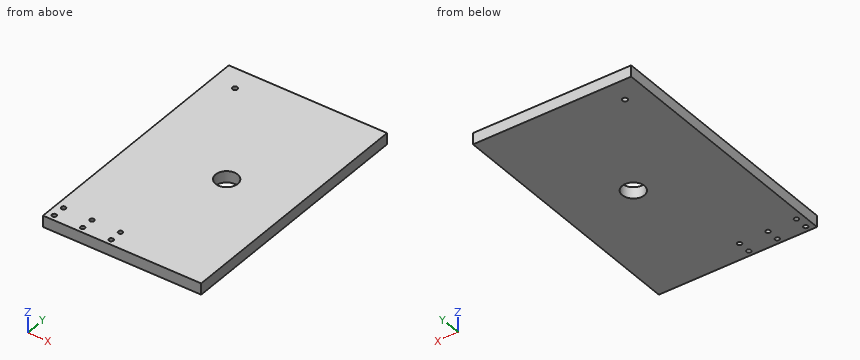
```python
from build123d import *

# Parameters (mm, degrees)
SKETCH1_W           = 152.4
SKETCH1_H           = 143.51
SKETCH1_R           = 6.223
SKETCH1_R_2         = 1.4375
BOSS_EXTRUDE1_DEPTH = 6.35
SKETCH2_R           = 3.1115
CUT_EXTRUDE1_DEPTH  = 105.859632486
SKETCH4_R           = 1.625
CUT_EXTRUDE2_DEPTH  = 105.859632486
SKETCH5_W           = 63.5
SKETCH5_H           = 143.51
CUT_EXTRUDE3_DEPTH  = 105.859632486
SKETCH6_R           = 1.25
CUT_EXTRUDE4_DEPTH  = 105.859632486


with BuildPart() as part:
    # Sketch1 → Boss-Extrude1 (new body)
    with BuildSketch(Plane.XY):
        Rectangle(SKETCH1_W, SKETCH1_H)
        with Locations((-25.272725174, 0.100300785)):
            Circle(SKETCH1_R, mode=Mode.SUBTRACT)
        with Locations((-63.5, 59.055)):
            Circle(SKETCH1_R_2, mode=Mode.SUBTRACT)
    extrude(amount=BOSS_EXTRUDE1_DEPTH)

    # Sketch2 → Cut-Extrude1 (cut, through all)
    with BuildSketch(Plane.XY.offset(6.35)):
        with Locations((63.5, 11.600300785)):
            Circle(SKETCH2_R)
    extrude(amount=-CUT_EXTRUDE1_DEPTH, mode=Mode.SUBTRACT)

    # Sketch4 → Cut-Extrude2 (cut, through all)
    with BuildSketch(Plane.XY.offset(6.35)):
        with Locations((43.849064669, -5.274915009)):
            Circle(SKETCH4_R)
        with Locations((43.849064669, -21.274915009)):
            Circle(SKETCH4_R)
        with Locations((43.849064669, -37.274915009)):
            Circle(SKETCH4_R)
        with Locations((43.849064669, 10.725084991)):
            Circle(SKETCH4_R)
    extrude(amount=-CUT_EXTRUDE2_DEPTH, mode=Mode.SUBTRACT)

    # Sketch5 → Cut-Extrude3 (cut, through all)
    with BuildSketch(Plane(origin=(0, 0, 0), x_dir=(-1, 0, 0), z_dir=(0, 0, -1))):
        with Locations((-44.45, 0)):
            Rectangle(SKETCH5_W, SKETCH5_H)
    extrude(amount=-CUT_EXTRUDE3_DEPTH, mode=Mode.SUBTRACT)

    # Sketch6 → Cut-Extrude4 (cut, through all)
    with BuildSketch(Plane(origin=(0, 0, 0), x_dir=(-1, 0, 0), z_dir=(0, 0, -1))):
        with Locations((72.2, -61.404999872)):
            Circle(SKETCH6_R)
        with Locations((56.2, -61.404999872)):
            Circle(SKETCH6_R)
        with Locations((40.2, -61.404999872)):
            Circle(SKETCH6_R)
        with Locations((72.2, -68.58)):
            Circle(SKETCH6_R)
        with Locations((56.2, -68.58)):
            Circle(SKETCH6_R)
        with Locations((40.2, -68.58)):
            Circle(SKETCH6_R)
    extrude(amount=-CUT_EXTRUDE4_DEPTH, mode=Mode.SUBTRACT)


solid = part.part
```
Work out the finished part from the listing and answer in its coordinate system (mm). Round coordinates to 2 decimals unless told otherwise and drop trailing zeros. Write each loop counter-clockwise with the first axis right and the second up, starting at its lowest first coordinate (ties: lowest second). Pieces come first, ordered by that corner, then holes. Notation, with made-up numbers: (1.25, -28.5) - (17.25, -28.5) arc R19 ccw to (17.25, 3.5) - close; hole circle Ø11 at (2, 57.25). An arc over 180 degrees is marked (long way). Return JSON: item names as keys, results as strings. Group by question number.
Q1. The part is cut by section A-A on x = -20.5. Write down the section's boundary in (y, z) (3 decimals), then the cut area to 3 significant figures.
Q2. Find the intervals of material crossed by L1, parallel to Y at x = -72.2, z = 4.25 (3 decimals); L2, parallel to X at y = -68.58, z = 3; L3, parallel to Y at x = -63.5, z = 3 (1 decimal), in increasing order.
Q3. This flat-tipped pin is pushed along its axis until it touches: pin 1 Ø4 at (x, y) = (-56.2, -68.58) entering from -Z. Where does it stop, or does it pass through?
Solved:
{
 "1": {"outline": "(-71.755, 0) - (-3.893, 0) - (-3.893, 6.35) - (-71.755, 6.35) - close; (4.094, 0) - (71.755, 0) - (71.755, 6.35) - (4.094, 6.35) - close", "area": "861 mm²"},
 "2": {"L1": "-71.755 to -69.83, -67.33 to -62.655, -60.155 to 71.755", "L2": "-76.2 to -73.45, -70.95 to -57.45, -54.95 to -41.45, -38.95 to 12.7", "L3": "-71.8 to 57.6, 60.5 to 71.8"},
 "3": {"pin 1": "z = 0"}
}
